```python
from build123d import *

# Parameters (mm, degrees)
SKETCH3_R           = 44.45
SKETCH3_R_2         = 38.1
BOSS_EXTRUDE3_DEPTH = 685.8
SKETCH4_W           = 63.5
SKETCH4_H           = 203.2
CUT_EXTRUDE2_DEPTH  = 685.8


with BuildPart() as part:
    # Sketch3 → Boss-Extrude3 (new body)
    with BuildSketch(Plane.XY):
        Circle(SKETCH3_R)
        Circle(SKETCH3_R_2, mode=Mode.SUBTRACT)
    extrude(amount=BOSS_EXTRUDE3_DEPTH)

    # Sketch4 → Cut-Extrude2 (cut)
    with BuildSketch(Plane(origin=(0, 0, 0), x_dir=(1, 0, 0), z_dir=(0, 1, 0))):
        with Locations((-0.892426947, -120.953055133)):
            Rectangle(SKETCH4_W, SKETCH4_H)
    extrude(amount=CUT_EXTRUDE2_DEPTH, mode=Mode.SUBTRACT)


solid = part.part
```
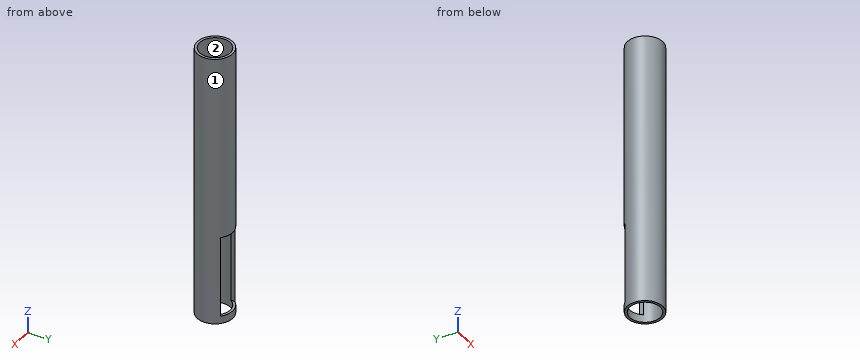
Design review of the part built by this model. Coordinates are the model's own, in mm. Face numbers are marked on the shaded views. Give positions to 0.01 mm unless a question says otherwise; leave off trailing zeros. Order: outer loops, then holes, each group sorted by start corner. A loop starts at its lowest first (then second) coordinate and runs counter-clockwise, first axis right, second up. Notation, with made-up numbers: (-10, -39) -> (4, -39) arc R15 cw to (4, -34) -> close; hole circle Ø4 at (14.25, 13.25). An arc over 180 degrees is marked (long way). Write each question's results on one line, items separated by ' | '. Start each with the question number.
Q1. For pin 1 (2 mm diameter, centred on y = -11.5, z = 82, fed in from -X); pin 2 (5 mm diameter, centred on y = -8, z = 182, fed in from -X); pin 3 (10.5 mm diameter, centred on y = 26.5, z = 103, fed in from -X); pin 4 (3 mm diameter, centred on x = 4.5, y = -35, fed in from +Z), all flat-tipped, find the tip position at first contact; note any pin that passes through.
Q2. Add section C-C on z = 508.5. Give the boundary of the cut face in (x, y), and give its area (3 significant figures).
Q3. Add section D-D on x = 9. Give the boundary of the cut face in (y, z).
Q4. Add section B-B on x = -19. Give the boundary of the cut face in (y, z).
Q5. Add section A-A on y = 0. Give the boundary of the cut face in (x, z), and give its area (3 significant figures).
Q6. Mouldability with a two-part tool opening along Y and no side actions: class the marked faces 1 and 2 as +Y half, -Y half, draft (parallel to the pull), parting line (faces both ways), or undercut.
Q7. Wall thickness on L1, parallel to Y at x = 0, z = 386; L2, parallel to Z at x = -21, y = 34; L3, parallel to X at y = -1.5, z = 336: over which ranges is each line inside the solid? List them lowest first. Write a range as from..to.
Found:
1) pin 1: stops at x = -43.19 | pin 2: stops at x = -44.11 | pin 3: stops at x = -39.04 | pin 4: passes through
2) outline: circle Ø88.9 at (0, 0); hole circle Ø76.2 at (0, 0) | area: 1,650 mm2
3) outline: (-43.53, 0) -> (-37.02, 0) -> (-37.02, 685.8) -> (-43.53, 685.8) -> close; (37.02, 0) -> (43.53, 0) -> (43.53, 19.35) -> (37.02, 19.35) -> close; (37.02, 222.55) -> (43.53, 222.55) -> (43.53, 685.8) -> (37.02, 685.8) -> close
4) outline: (-40.18, 0) -> (-33.02, 0) -> (-33.02, 685.8) -> (-40.18, 685.8) -> close; (33.02, 0) -> (40.18, 0) -> (40.18, 19.35) -> (33.02, 19.35) -> close; (33.02, 222.55) -> (40.18, 222.55) -> (40.18, 685.8) -> (33.02, 685.8) -> close
5) outline: (-44.45, 0) -> (-38.1, 0) -> (-38.1, 685.8) -> (-44.45, 685.8) -> close; (38.1, 0) -> (44.45, 0) -> (44.45, 685.8) -> (38.1, 685.8) -> close | area: 8,710 mm2
6) face 1: parting line | face 2: undercut
7) L1: y = -44.45..-38.1, 38.1..44.45 | L2: z = 0..19.35, 222.55..685.8 | L3: x = -44.42..-38.07, 38.07..44.42
